For this review, take the finished solid that the model builds, in its own axes (mm). Round coordinates to 2 decimals unless told otherwise and drop trailing zeros. Order: outer loops, then holes, each group sorted by start corner. A loop starts at its lowest first (then second) coordinate and runs counter-clockwise, first axis right, second up. Notation, with made-up numbers: (72.25, 31) - (83.25, 31) arc R33 cw to (83.25, 65) - close; hole circle Ø5 at (20.5, 28.5). An arc over 180 degrees is marked (long way). One line per question, with ' | ' between items.
```python
from build123d import *

# Parameters (mm, degrees)
SKETCH1_W           = 81.534
SKETCH1_H           = 104.902
BOSS_EXTRUDE1_DEPTH = 1.524
SKETCH2_W           = 9.17
SKETCH2_H           = 5.95
SKETCH2_W_2         = 9.266089767
SKETCH2_H_2         = 5.472
CUT_EXTRUDE1_DEPTH  = 1.524
SKETCH4_W           = 56.5
SKETCH4_H           = 17
CUT_EXTRUDE2_DEPTH  = 1.524
SKETCH6_R           = 2.285
CUT_EXTRUDE3_DEPTH  = 1.524
SKETCH8_R           = 8.224077239
CUT_EXTRUDE4_DEPTH  = 2.54


with BuildPart() as part:
    # Sketch1 → Boss-Extrude1 (new body)
    with BuildSketch(Plane.XY):
        with Locations((-2.046973799, -6.087681223)):
            Rectangle(SKETCH1_W, SKETCH1_H)
    extrude(amount=BOSS_EXTRUDE1_DEPTH)

    # Sketch2 → Cut-Extrude1 (cut)
    with BuildSketch(Plane.XY.offset(1.524)):
        with Locations((-38.228973799, -55.563681223)):
            Rectangle(SKETCH2_W, SKETCH2_H)
        with Locations((34.086981318, -55.802681223)):
            Rectangle(SKETCH2_W_2, SKETCH2_H_2)
    extrude(amount=-CUT_EXTRUDE1_DEPTH, mode=Mode.SUBTRACT)

    # Sketch4 → Cut-Extrude2 (cut)
    with BuildSketch(Plane.XY.offset(1.524)):
        with Locations((-6.933973799, -38.698681223)):
            Rectangle(SKETCH4_W, SKETCH4_H)
    extrude(amount=-CUT_EXTRUDE2_DEPTH, mode=Mode.SUBTRACT)

    # Sketch6 → Cut-Extrude3 (cut)
    with BuildSketch(Plane.XY.offset(1.524)):
        with Locations((-2.046973799, 40.158318777)):
            Circle(SKETCH6_R)
        with Locations((34.265026201, 37.193318777)):
            Circle(SKETCH6_R)
    extrude(amount=-CUT_EXTRUDE3_DEPTH, mode=Mode.SUBTRACT)

    # Sketch8 → Cut-Extrude4 (cut)
    with BuildSketch(Plane.XY.offset(1.524)):
        with Locations((-7.753098943, 30.457244975)):
            Circle(SKETCH8_R)
    extrude(amount=-CUT_EXTRUDE4_DEPTH, mode=Mode.SUBTRACT)


solid = part.part
```
(1) We need section A-A on x = 9. State the section outline as (y, z) points, plus the area to 3 significant figures.
Output values:
outline: (-58.54, 0) - (-47.2, 0) - (-47.2, 1.52) - (-58.54, 1.52) - close; (-30.2, 0) - (46.36, 0) - (46.36, 1.52) - (-30.2, 1.52) - close | area: 134 mm^2
(2) For probe 1 along X at (y, z) = (-39, 0.4); probe 2 along Y at (x, z) = (-30, 0.85); probe 3 along Y at (x, z) = (-7, 0.3), list the stretches that pass through material, from the lowest coordinate up. Write a range as [from, to].
Output values:
probe 1: [-42.81, -35.18], [21.32, 38.72] | probe 2: [-58.54, -47.2], [-30.2, 46.36] | probe 3: [-58.54, -47.2], [-30.2, 22.27], [38.65, 46.36]
(3) We need section C-C on x = -8.5. State the section outline as (y, z) points.
Output values:
outline: (-58.54, 0) - (-47.2, 0) - (-47.2, 1.52) - (-58.54, 1.52) - close; (-30.2, 0) - (22.27, 0) - (22.27, 1.52) - (-30.2, 1.52) - close; (38.65, 0) - (46.36, 0) - (46.36, 1.52) - (38.65, 1.52) - close
(4) Mouldability with a two-part tool opening along X and no side actions: class faces 1 (the flat face through (-3, -5, 1.524)), 2 (the cylindrical face through (-2.344, 42.424, 0.773)), 3 (the cylindrical face through (-3.33, 37.39, 0.77)) as released by +X, released by -X, zero draft, split by the parting line, or undercut.
Output values:
face 1: zero draft | face 2: undercut | face 3: undercut
(5) We need section B-B on y = 33. State the section outline as (x, z) points.
Output values:
outline: (-42.81, 0) - (-15.57, 0) - (-15.57, 1.52) - (-42.81, 1.52) - close; (0.07, 0) - (38.72, 0) - (38.72, 1.52) - (0.07, 1.52) - close
(6) Insertion check: pin 1 (0.8 mm diameter, centred on y = -55.5, z = 1, fed in from -X); pin 2 (0.5 mm diameter, centred on x = -38.5, z = 1, fed in from -Y); pin 3 (0.5 mm diameter, centred on x = 33.5, z = 0.5, fed in from -Y). Each pin has a flat end and moves straight along its axis. Give the tip position at first contact, or say it passes through.
Output values:
pin 1: x = -33.64 | pin 2: y = -52.59 | pin 3: y = -53.07
(7) We need section D-D on z = 0.95. State the section outline as (x, y) points (3 decimals).
Output values:
outline: (-42.814, -52.589) - (-33.644, -52.589) - (-33.644, -58.539) - (29.454, -58.539) - (29.454, -53.067) - (38.72, -53.067) - (38.72, 46.363) - (-42.814, 46.363) - close; hole (-35.184, -47.199) - (21.316, -47.199) - (21.316, -30.199) - (-35.184, -30.199) - close; hole circle Ø16.448 at (-7.753, 30.457); hole circle Ø4.57 at (-2.047, 40.158); hole circle Ø4.57 at (34.265, 37.193)
